Read the model definition and answer for the solid it produces. Units are mm, in the model's axes. Face numbers are marked on the shaded views. A direction names the side the tool comes from. Give positions to 0.01 mm unless a question says otherwise; leave off trailing zeros. Write each question's results on one line, items separated by ' | '.
from build123d import *

# Parameters (mm, degrees)
SKETCH1_R           = 37.5
BOSS_EXTRUDE1_DEPTH = 10
BOSS_EXTRUDE2_DEPTH = 15
SKETCH8_R           = 0.75
CUT_EXTRUDE1_DEPTH  = 11


with BuildPart() as part:
    # Sketch1 → Boss-Extrude1 (new body)
    with BuildSketch(Plane(origin=(0, 0, 0), x_dir=(1, 0, 0), z_dir=(0, 1, 0))):
        Circle(SKETCH1_R)
    extrude(amount=BOSS_EXTRUDE1_DEPTH)

    # Sketch5 → Revolve1 (revolve)
    with BuildSketch(Plane(origin=(0, 0, 0), x_dir=(0, 0, -1), z_dir=(1, 0, 0))):
        with BuildLine():
            Line((-37.5, 25), (-37.5, 10))
            Line((-37.5, 10), (-22.5, 10))
            add(Edge.make_bspline(
                [(-37.5, 25), (-36.468402779, 11.405172281), (-22.5, 10)],
                knots=[0, 0, 0, 1, 1, 1], degree=2))
        make_face()
    revolve(axis=Axis((0, 0, 0), (0, 1, 0)))

    # Sketch7 → Boss-Extrude2 (add)
    with BuildSketch(Plane(origin=(0, 10, 0), x_dir=(1, 0, 0), z_dir=(0, 1, 0))):
        with BuildLine():
            Line((36.742346142, 7.5), (7.5, 7.5))
            Line((7.5, 7.5), (7.5, 36.742346142))
            ThreePointArc((7.5, 36.742346142), (0, 37.5), (-7.5, 36.742346142))
            Line((-7.5, 36.742346142), (-7.5, 7.5))
            Line((-7.5, 7.5), (-36.742346142, 7.5))
            ThreePointArc((-36.742346142, 7.5), (-37.5, 0), (-36.742346142, -7.5))
            Line((-36.742346142, -7.5), (-7.5, -7.5))
            Line((-7.5, -7.5), (-7.5, -36.742346142))
            ThreePointArc((-7.5, -36.742346142), (0, -37.5), (7.5, -36.742346142))
            Line((7.5, -36.742346142), (7.5, -7.5))
            Line((7.5, -7.5), (36.742346142, -7.5))
            ThreePointArc((36.742346142, -7.5), (37.5, 0), (36.742346142, 7.5))
        make_face()
    extrude(amount=BOSS_EXTRUDE2_DEPTH)

    # Sketch8 → Cut-Extrude1 (cut, through all)
    with BuildSketch(Plane(origin=(0, 10, 0), x_dir=(1, 0, 0), z_dir=(0, 1, 0))):
        with Locations((-10.50286976, 10.50286976)):
            Circle(SKETCH8_R)
        with Locations((-12.907032816, 12.907032816)):
            Circle(SKETCH8_R)
        with Locations((10.50286976, 10.50286976)):
            Circle(SKETCH8_R)
        with Locations((12.907032816, 12.907032816)):
            Circle(SKETCH8_R)
        with Locations((10.50286976, -10.50286976)):
            Circle(SKETCH8_R)
        with Locations((12.907032816, -12.907032816)):
            Circle(SKETCH8_R)
        with Locations((-10.50286976, -10.50286976)):
            Circle(SKETCH8_R)
        with Locations((-12.907032816, -12.907032816)):
            Circle(SKETCH8_R)
    extrude(amount=-CUT_EXTRUDE1_DEPTH, mode=Mode.SUBTRACT)


solid = part.part
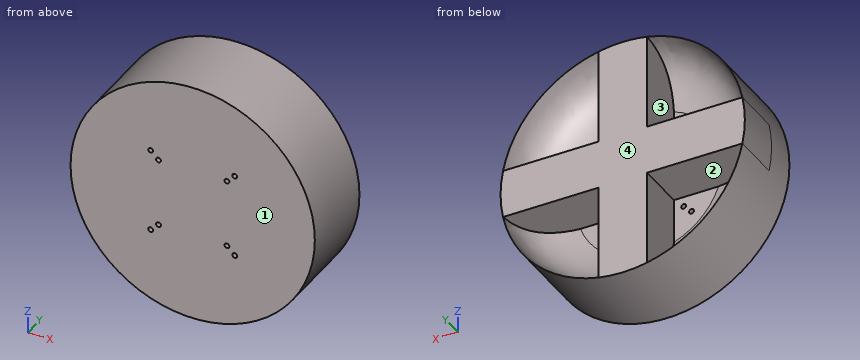
(1) Consider probe 1 along X at (y, z) = (13.25, -11.5); probe 2 along X at (y, z) = (20, -32); probe 3 along Z at (x, y) = (27.5, 16.5). Determine where each line is inside the solid, lowest interval first. Write a range as [from, to].
Conclusion:
probe 1: [-35.69, -29.7], [-7.5, 7.5], [29.7, 35.69] | probe 2: [-19.55, -17.67], [-7.5, 7.5], [17.67, 19.55] | probe 3: [-25.5, -21.48], [-7.5, 7.5], [21.48, 25.5]
(2) For the marked faces 3 and 4, determine the directions among +Z, -Z, +X, -X, +Y, -Y from which every point of the face is accessible in a straight line to the end or side of a thin tool.
Conclusion:
face 3: +Y | face 4: +Z, -Z, +X, -X, +Y
(3) Section A-A (y = 5.5) is taken. State how many separate pieces and enclosed holes the cut face has, plus the area to 3 significant figures.
Conclusion:
separate pieces: 1 | enclosed holes: 8 | area: 4,400 mm^2
(4) Each of these flat-tipped pins is pushed along its axis until it touches: pin 1 (1 mm diameter, centred on x = -21.5, y = 21.5, fed in from +Z); pin 2 (7.5 mm diameter, centred on y = 14, z = -28, fed in from +X); pin 3 (10 mm diameter, centred on y = 13.5, z = -13, fed in from -X); pin 4 (0.9 mm diameter, centred on x = -12.91, z = 12.91, fed in from -Y). Where does it stop, or does it pass through?
Conclusion:
pin 1: z = 31.07 | pin 2: x = 28.6 | pin 3: x = -36.64 | pin 4: through
(5) The mould has two halves that part along X. Classify the marked faces 1 and 2: pulls with the +X half, pulls with the -X half, needs draft (parallel to the pull), parting line crosses it, or undercut.
Conclusion:
face 1: needs draft | face 2: undercut
